```python
from build123d import *

# Parameters (mm, degrees)
SKETCH1_R           = 3
BOSS_EXTRUDE1_DEPTH = 2
FILLET1_R           = 5


with BuildPart() as part:
    # Sketch1 → Boss-Extrude1 (new body)
    with BuildSketch(Plane.XY):
        with BuildLine():
            Line((-17.5, -29.9861237), (-33.570384709, -29.9861237))
            Line((-33.570384709, -29.9861237), (-33.570384709, 7.191652864))
            ThreePointArc((-33.570384709, 7.191652864), (-35.102603086, 12.763157514), (-39.268321068, 16.767673829))
            Line((-39.268321068, 16.767673829), (-53.500564058, 24.492870138))
            ThreePointArc((-53.500564058, 24.492870138), (0, 58.627853025), (53.500564058, 24.492870138))
            Line((53.500564058, 24.492870138), (39.268321068, 16.767673829))
            ThreePointArc((39.268321068, 16.767673829), (35.102603086, 12.763157514), (33.570384709, 7.191652864))
            Line((33.570384709, 7.191652864), (33.570384709, -29.9861237))
            Line((33.570384709, -29.9861237), (17.5, -29.9861237))
            Line((17.5, -29.9861237), (17.5, -0.731973174))
            ThreePointArc((17.5, -0.731973174), (0, 17.137840029), (-17.5, -0.731973174))
            Line((-17.5, -0.731973174), (-17.5, -29.9861237))
        make_face()
        with Locations((-25, -12.5)):
            Circle(SKETCH1_R, mode=Mode.SUBTRACT)
        with Locations((25, -12.5)):
            Circle(SKETCH1_R, mode=Mode.SUBTRACT)
        Polygon((-35.777618692, 17.865360065), (-30.408261188, 14.765360065), (-29.308261188, 16.670615954), (-34.677618692, 19.770615954), align=None, mode=Mode.SUBTRACT)
        Polygon((30.408261188, 14.765360065), (29.308261188, 16.670615954), (34.677618692, 19.770615954), (35.777618692, 17.865360065), align=None, mode=Mode.SUBTRACT)
    extrude(amount=BOSS_EXTRUDE1_DEPTH)

    # Fillet1
    fillet1_edges = [part.edges().sort_by_distance(p)[0] for p in [
        (-53.500564058, 24.492870138, 1),
        (53.500564058, 24.492870138, 1),
    ]]
    fillet(fillet1_edges, radius=FILLET1_R)


solid = part.part
```
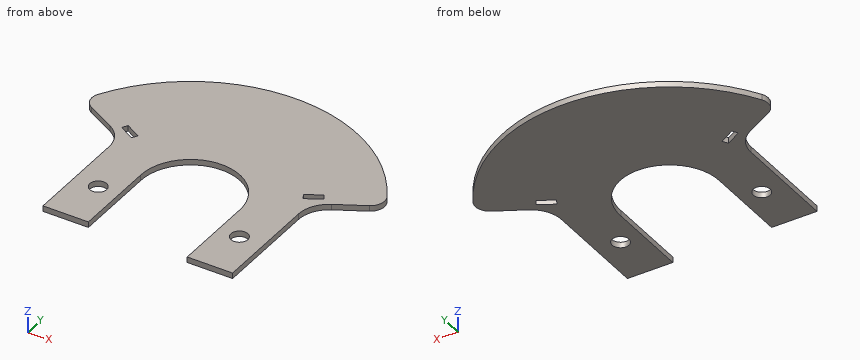
The model under review builds one solid part; all positions refer to its coordinate system, in mm. Round coordinates to 2 decimals unless told otherwise and drop trailing zeros. Write each loop counter-clockwise with the first axis right and the second up, starting at its lowest first coordinate (ties: lowest second). Pieces come first, ordered by that corner, then holes. Notation, with made-up numbers: M 66.25,-7 L 106.25,-7 A8 cw 106.25,7 Z; hole C 25.5,68 d10. An arc over 180 degrees is marked long. Use CSV: the item, a comma, the result in double quotes. Start each with the question number.
(1) Clearance check with flat-ended pins moving along their axes: P1, Ø1, axis at y = -19, z = 1, coming from the +X side; P2, Ø4, axis at x = 31.5, y = -13, coming from the -Z side; P3, Ø5.5, axis at x = 25, y = -12.5, coming from the -Z side; P4, Ø1, axis at x = 14.5, z = 1, coming from the -Y side. State where each tip first meets the part, or that it passes through.
(2) We need section C-C, the plane z = 1.7. State the section outline as (x, y) points.
(3) For line 1 along Y through (x, z) = (-35.5, 1.05); line 2 along Y through (x, z) = (-25, 1.5); line 3 along X through (y, z) = (2.5, 0.25), list the stretches that pass through material, from the lowest coordinate up.
(4) We need section B-B, the plane x = -25. State the section outline as (y, z) points, then the cut area to 3 significant figures.
(5) We need section D-D, the plane x = 0. State the section outline as (y, z) points, then the cut area to 3 significant figures.
(6) We need section A-A, the plane y = -12.5. State the section outline as (x, z) points, then the cut area to 3 significant figures.
Findings:
1,P1,"x = 33.57"
1,P2,"z = 0"
1,P3,"through"
1,P4,"y = 8.66"
2,outline,"M -51.14,29.04 A5 ccw -49.19,22.15 L -39.27,16.77 A10.9 cw -33.57,7.19 L -33.57,-29.99 L -17.5,-29.99 L -17.5,-0.73 A17.5 cw long 17.5,-0.73 L 17.5,-29.99 L 33.57,-29.99 L 33.57,7.19 A10.9 cw 39.27,16.77 L 49.19,22.15 A5 ccw 51.14,29.04 A58.99 ccw Z; hole M -35.78,17.87 L -30.41,14.77 L -29.31,16.67 L -34.68,19.77 Z; hole C -25,-12.5 d6; hole C 25,-12.5 d6; hole M 29.31,16.67 L 30.41,14.77 L 35.78,17.87 L 34.68,19.77 Z"
3,line 1,"13.38 to 17.71, 18.35 to 46.75"
3,line 2,"-29.99 to -15.5, -9.5 to 53.07"
3,line 3,"-33.57 to -17.27, 17.27 to 33.57"
4,outline,"M -29.99,0 L -15.5,0 L -15.5,2 L -29.99,2 Z; M -9.5,0 L 53.07,0 L 53.07,2 L -9.5,2 Z"
4,area,"154 mm^2"
5,outline,"M 17.14,0 L 58.63,0 L 58.63,2 L 17.14,2 Z"
5,area,"83.0 mm^2"
6,outline,"M -33.57,0 L -28,0 L -28,2 L -33.57,2 Z; M -22,0 L -17.5,0 L -17.5,2 L -22,2 Z; M 17.5,0 L 22,0 L 22,2 L 17.5,2 Z; M 28,0 L 33.57,0 L 33.57,2 L 28,2 Z"
6,area,"40.3 mm^2"
